from build123d import *

# Parameters (mm, degrees)
PAD_DEPTH       = 12
SKETCH001_R     = 1.6
POCKET_DEPTH    = 6.001
SKETCH002_W     = 0.9
SKETCH002_H     = 0.9
POCKET001_DEPTH = 12.001
SKETCH003_W     = 0.9
SKETCH003_H     = 1.5
POCKET002_DEPTH = 4.901
FILLET_R        = 1
PAD001_DEPTH    = 6
FILLET001_R     = 1
CHAMFER_SIZE    = 1
CHAMFER001_SIZE = 0.4


with BuildPart() as part:
    # Sketch → Pad (new body)
    with BuildSketch(Plane.XY):
        Polygon((-14.25, 0), (-9, 0), (-9, -3), (9, -3), (9, 0), (14.25, 0), (14.25, 6), (-14.25, 6), align=None)
    extrude(amount=PAD_DEPTH)

    # Sketch001 → Pocket (cut, through all)
    with BuildSketch(Plane.XZ):
        with Locations((-12, 7.5)):
            Circle(SKETCH001_R)
        with Locations((12, 7.5)):
            Circle(SKETCH001_R)
    extrude(amount=-POCKET_DEPTH, mode=Mode.SUBTRACT)

    # Sketch002 → Pocket001 (cut, through all)
    with BuildSketch(Plane.XY):
        with Locations((-3.81, 0.65)):
            Rectangle(SKETCH002_W, SKETCH002_H)
        with Locations((3.81, 0.65)):
            Rectangle(SKETCH002_W, SKETCH002_H)
    extrude(amount=POCKET001_DEPTH, mode=Mode.SUBTRACT)

    # Sketch003 (on Face15 of Pocket001) → Pocket002 (cut, through all)
    with BuildSketch(Plane.XZ.offset(-1.1)):
        with Locations((3.81, 11.25)):
            Rectangle(SKETCH003_W, SKETCH003_H)
        with Locations((-3.81, 11.25)):
            Rectangle(SKETCH003_W, SKETCH003_H)
    extrude(amount=-POCKET002_DEPTH, mode=Mode.SUBTRACT)

    # Fillet
    fillet_edges = [part.edges().sort_by_distance(p)[0] for p in [
        (3.81, 1.1, 10.5),
        (-3.81, 1.1, 10.5),
    ]]
    fillet(fillet_edges, radius=FILLET_R)

    # Sketch004 → Pad001 (join)
    with BuildSketch(Plane.XZ):
        with BuildLine():
            ThreePointArc((14.25, 5.918861), (14.75, 7.5), (14.25, 9.081139))
            Line((14.25, 9.081139), (14.25, 5.918861))
        make_face()
    pad001 = extrude(amount=-PAD001_DEPTH)

    # Mirrored: Pad001 across Sketch004 V_Axis
    add(pad001.mirror(Plane(origin=(0, 0, 0), x_dir=(0, -1, 0), z_dir=(1, 0, 0))))

    # Fillet001
    fillet001_edges = [part.edges().sort_by_distance(p)[0] for p in [
        (14.25, 3, 9.081139),
        (14.25, 3, 5.918861),
        (-14.25, 3, 9.081139),
        (-14.25, 3, 5.918861),
    ]]
    fillet(fillet001_edges, radius=FILLET001_R)

    # Chamfer
    chamfer_edges = [part.edges().sort_by_distance(p)[0] for p in [
        (14.25, 3, 12),
        (-14.25, 3, 12),
        (9, -3, 6),
        (-9, -3, 6),
    ]]
    chamfer(chamfer_edges, length=CHAMFER_SIZE)

    # Chamfer001
    chamfer001_edges = [part.edges().sort_by_distance(p)[0] for p in [
        (-9, -1, 0),
        (-8.5, -2.5, 0),
        (-11.625, 0, 0),
        (0, -3, 0),
        (-14.25, 3, 0),
        (8.5, -2.5, 0),
        (0, 6, 0),
        (9, -1, 0),
        (14.25, 3, 0),
        (11.625, 0, 0),
        (3.36, 0.65, 0),
        (3.81, 0.2, 0),
        (4.26, 0.65, 0),
        (3.81, 1.1, 0),
        (-4.26, 0.65, 0),
        (-3.81, 0.2, 0),
        (-3.36, 0.65, 0),
        (-3.81, 1.1, 0),
    ]]
    chamfer(chamfer001_edges, length=CHAMFER001_SIZE)


solid = part.part
Could you check a few things on this model? Use its own coordinates, in mm. A direction names the side the tool comes from. Coordinates: 2 decimals unless noted, no trailing zeros. Write each loop counter-clockwise with the first axis right and the second up, starting at its lowest first coordinate (ties: lowest second). Pieces come first, ordered by that corner, then holes. Notation, with made-up numbers: (40, 3.5) - (87, 3.5) arc R10 cw to (87, 17.5) - close; hole circle Ø9 at (82, -22.75). An arc over 180 degrees is marked (long way). Put each result on its own line as item: value. Start each with the question number.
Q1. I want a section at C-C on y = 4. Write out the boundary of the cut face in (x, z).
Q2. I want a section at B-B on x = -12. Write out the boundary of the cut face in (y, z), plus the area to 3 significant figures.
Q3. I want a section at A-A on z = 7.5. Write out the boundary of the cut face in (x, y).
Q4. Please list where these lines run through material, in increasing order: L1, parallel to X at y = 0.75, z = 9.75; L2, parallel to Y at x = 4, z = 4; L3, parallel to Z at x = -12, y = 1.75.
Q5. Thinking about a two-plate mould opening in X: for faces 1 (the flat face through (4.26, 0.9, 8.3)), 2 (the flat face through (14.25, 3, 10)), 3 (the flat face through (11, 0, 6)), 4 (the flat face through (-8.5, -2.5, 6.1)), which applies, pulls with the +X half, pulls with the -X half, needs draft (parallel to the pull), parting line crosses it, or undercut?
Q6. Which directions (+Z, -Z, +X, -X, +Y, -Y) give clear straight access to the entire face, cutting with the end or side of a thin tool? Please do faces 5 (the flat face through (9, -1, 6)), 6 (the flat face through (14.25, 3, 3)), 7 (the flat face through (-9, -1, 6)), 8 (the flat face through (4, 4, 10.5)), 9 (the flat face through (-14.25, 3, 10)).
Q7. I want a section at D-D on z = 2.75. Write out the boundary of the cut face in (x, y).
Q8. I'm going to push flat-ended pins straight in: P1, Ø1.6, axis at y = 1.5, z = 1.5, coming from the -X side; P2, Ø3.5, axis at x = -12, z = 7.5, coming from the -Y side; P3, Ø0.6, axis at y = -1.5, z = 4.5, coming from the +X side; P4, Ø2.5, axis at x = 12, z = 7.5, coming from the -Y side. Where does each tip first touch, or does it pass through?
Checks:
1. outline: (-14.38, 6.13) arc R1 cw to (-14.25, 5.63) - (-14.25, 0.4) - (-13.85, 0) - (13.85, 0) - (14.25, 0.4) - (14.25, 5.63) arc R1 cw to (14.38, 6.13) arc R2.75 ccw to (14.38, 8.87) arc R1 cw to (14.25, 9.37) - (14.25, 11) - (13.25, 12) - (4.26, 12) - (4.26, 10.5) - (3.36, 10.5) - (3.36, 12) - (-3.36, 12) - (-3.36, 10.5) - (-4.26, 10.5) - (-4.26, 12) - (-13.25, 12) - (-14.25, 11) - (-14.25, 9.37) arc R1 cw to (-14.38, 8.87) arc R2.75 ccw to start; hole circle Ø3.2 at (-12, 7.5); hole circle Ø3.2 at (12, 7.5)
2. outline: (0, 0.4) - (0.4, 0) - (5.6, 0) - (6, 0.4) - (6, 5.9) - (0, 5.9) - close; (0, 9.1) - (6, 9.1) - (6, 12) - (0, 12) - close
2. area: 52.6 mm²
3. outline: (-14.75, 0) - (-13.6, 0) - (-13.6, 6) - (-14.75, 6) - close; (-10.4, 0) - (-9, 0) - (-9, -2) - (-8, -3) - (8, -3) - (9, -2) - (9, 0) - (10.4, 0) - (10.4, 6) - (-10.4, 6) - close; (13.6, 0) - (14.75, 0) - (14.75, 6) - (13.6, 6) - close; hole (-4.26, 0.2) - (-3.36, 0.2) - (-3.36, 1.1) - (-4.26, 1.1) - close; hole (3.36, 0.2) - (4.26, 0.2) - (4.26, 1.1) - (3.36, 1.1) - close
4. L1: -14.25 to -4.26, -3.36 to 3.36, 4.26 to 14.25
4. L2: -3 to 0.2, 1.1 to 6
4. L3: 0 to 5.9, 9.1 to 12
5. face 1: undercut
5. face 2: pulls with the +X half
5. face 3: needs draft
5. face 4: pulls with the -X half
6. face 5: +Z, -Z, +X, -Y
6. face 6: -Z, +X, +Y, -Y
6. face 7: +Z, -Z, -X, -Y
6. face 8: +Z, +Y
6. face 9: +Z, -X, +Y, -Y
7. outline: (-14.25, 0) - (-9, 0) - (-9, -2) - (-8, -3) - (8, -3) - (9, -2) - (9, 0) - (14.25, 0) - (14.25, 6) - (-14.25, 6) - close; hole (-4.26, 0.2) - (-3.36, 0.2) - (-3.36, 1.1) - (-4.26, 1.1) - close; hole (3.36, 0.2) - (4.26, 0.2) - (4.26, 1.1) - (3.36, 1.1) - close
8. P1: x = -14.25
8. P2: y = 0
8. P3: x = 9
8. P4: through
